from build123d import *

# Parameters (mm, degrees)
BOSS_EXTRUDE1_DEPTH  = 6
SKETCH3_W            = 26.265732208
SKETCH3_H            = 53.5
CUT_EXTRUDE2_DEPTH   = 6
BOSS_EXTRUDE2_DEPTH  = 3.175
CUT_EXTRUDE3_DEPTH   = 9.175
SKETCH5_W            = 6.5
SKETCH5_H            = 3
CUT_EXTRUDE4_DEPTH   = 6.95
SKETCH6_R            = 2.5
CUT_EXTRUDE5_DEPTH   = 10
M3_CLEARANCE_HOLE1_D = 3.2
SKETCH17_R           = 41
BOSS_EXTRUDE3_DEPTH  = 10
SKETCH18_R           = 2.5
CUT_EXTRUDE6_DEPTH   = 5
SKETCH19_R           = 4.5
CUT_EXTRUDE7_DEPTH   = 11.5
SKETCH20_R           = 2.706261539
SKETCH20_R_2         = 3.316969597
CUT_EXTRUDE8_DEPTH   = 6


with BuildPart() as part:
    # Sketch1 → Boss-Extrude1 (new body)
    with BuildSketch(Plane(origin=(0, 0, 0), x_dir=(1, 0, 0), z_dir=(0, 1, 0))):
        with BuildLine():
            Line((-21.25, 28.5), (-21.25, -28.5))
            ThreePointArc((-21.25, -28.5), (0, -33.5), (21.25, -28.5))
            Line((21.25, -28.5), (21.25, 28.5))
            Line((21.25, 28.5), (-21.25, 28.5))
        make_face()
        with BuildLine():
            Line((-17.45, 32), (-17.45, 28.5))
            Line((-17.45, 28.5), (17.45, 28.5))
            Line((17.45, 28.5), (17.45, 32))
            ThreePointArc((17.45, 32), (0, 37.8), (-17.45, 32))
        make_face()
    extrude(amount=BOSS_EXTRUDE1_DEPTH)

    # Sketch3 → Cut-Extrude2 (cut)
    with BuildSketch(Plane.XZ):
        with Locations((-30.582866104, -1.75)):
            Rectangle(SKETCH3_W, SKETCH3_H)
        with Locations((30.582866104, -1.75)):
            Rectangle(SKETCH3_W, SKETCH3_H)
    extrude(amount=-CUT_EXTRUDE2_DEPTH, mode=Mode.SUBTRACT)

    # Sketch2 → Boss-Extrude2 (add)
    with BuildSketch(Plane(origin=(0, 6, 0), x_dir=(1, 0, 0), z_dir=(0, 1, 0))):
        with BuildLine():
            Line((-7.375, 17.3), (-7.375, 37.8))
            Line((-7.375, 37.8), (7.375, 37.8))
            Line((7.375, 37.8), (7.375, 17.3))
            ThreePointArc((7.375, 17.3), (0, 12.5), (-7.375, 17.3))
        make_face()
    extrude(amount=BOSS_EXTRUDE2_DEPTH)

    # Sketch4 → Cut-Extrude3 (cut)
    with BuildSketch(Plane.XZ):
        with BuildLine():
            Line((17.45, -32), (17.45, -50.042511561))
            Line((17.45, -50.042511561), (-17.45, -50.042511561))
            Line((-17.45, -50.042511561), (-17.45, -32))
            ThreePointArc((-17.45, -32), (0, -37.8), (17.45, -32))
        make_face()
    extrude(amount=-CUT_EXTRUDE3_DEPTH, mode=Mode.SUBTRACT)

    # Sketch5 → Cut-Extrude4 (cut)
    with BuildSketch(Plane(origin=(0, 9.175, 0), x_dir=(1, 0, 0), z_dir=(0, 1, 0))):
        with Locations((0, 31.3)):
            Rectangle(SKETCH5_W, SKETCH5_H)
    extrude(amount=-CUT_EXTRUDE4_DEPTH, mode=Mode.SUBTRACT)

    # Sketch6 → Cut-Extrude5 (cut)
    with BuildSketch(Plane(origin=(0, 9.175, -37.8), x_dir=(-1, 0, 0), z_dir=(0, 0, -1))):
        with Locations((0, -4.2)):
            Circle(SKETCH6_R)
    extrude(amount=-CUT_EXTRUDE5_DEPTH, mode=Mode.SUBTRACT)

    # M3 Clearance Hole1 (through all)
    with Locations(Plane(origin=(0, 0, 0), x_dir=(-1, 0, 0), z_dir=(0, -1, 0))):
        with Locations((0, 2.15)):
            Hole(M3_CLEARANCE_HOLE1_D / 2)

    # Sketch17 → Boss-Extrude3 (add)
    with BuildSketch(Plane.XZ):
        with Locations((0, -2.15)):
            Circle(SKETCH17_R)
    extrude(amount=BOSS_EXTRUDE3_DEPTH)

    # Sketch18 → Cut-Extrude6 (cut)
    with BuildSketch(Plane.XZ.offset(10)):
        with Locations((17.78, -32.945863359)):
            Circle(SKETCH18_R)
        with Locations((35.56, -2.15)):
            Circle(SKETCH18_R)
        with Locations((17.78, 28.645863359)):
            Circle(SKETCH18_R)
        with Locations((-17.78, -32.945863359)):
            Circle(SKETCH18_R)
        with Locations((-35.56, -2.15)):
            Circle(SKETCH18_R)
        with Locations((-17.78, 28.645863359)):
            Circle(SKETCH18_R)
    extrude(amount=-CUT_EXTRUDE6_DEPTH, mode=Mode.SUBTRACT)

    # Sketch19 → Cut-Extrude7 (cut)
    with BuildSketch(Plane(origin=(0, 6, 0), x_dir=(1, 0, 0), z_dir=(0, 1, 0))):
        with Locations((-17.78, 32.945863359)):
            Circle(SKETCH19_R)
        with Locations((17.78, 32.945863359)):
            Circle(SKETCH19_R)
        with Locations((35.56, 2.15)):
            Circle(SKETCH19_R)
        with Locations((17.78, -28.645863359)):
            Circle(SKETCH19_R)
        with Locations((-17.78, -28.645863359)):
            Circle(SKETCH19_R)
        with Locations((-35.56, 2.15)):
            Circle(SKETCH19_R)
    extrude(amount=-CUT_EXTRUDE7_DEPTH, mode=Mode.SUBTRACT)

    # Sketch20 → Cut-Extrude8 (cut)
    with BuildSketch(Plane(origin=(0, 6, 0), x_dir=(1, 0, 0), z_dir=(0, 1, 0))):
        with Locations((-20.581445068, -26.580263628)):
            Circle(SKETCH20_R)
        with Locations((20.21362745, -26.580263628)):
            Circle(SKETCH20_R_2)
    extrude(amount=-CUT_EXTRUDE8_DEPTH, mode=Mode.SUBTRACT)


solid = part.part
Input: part model. Units: mm. Frame: model coordinates. A direction names the side the tool comes from. Coordinates: 2 decimals unless noted, no trailing zeros. Order: outer loops, then holes, each group sorted by start corner. A loop starts at its lowest first (then second) coordinate and runs counter-clockwise, first axis right, second up. Notation, with made-up numbers: M 72,4 L 94,4 A19 cw 94,34 Z; hole C 50.5,4 d11. An arc over 180 degrees is marked long. One line per question, with ' | ' between items.
Item 1: Section D-D (y = -1.25). Output: boundary loops of the cut face in (x, z), then the cut area to 3 significant figures.
Geometry results:
outline: C 0,-2.15 d82; hole C -35.56,-2.15 d9; hole C -17.78,-32.95 d9; hole C -17.78,28.65 d9; hole C 17.78,-32.95 d9; hole C 17.78,28.65 d9; hole C 35.56,-2.15 d9 | area: 4,900 mm^2
Item 2: Section A-A (z = -2.15). Output: boundary loops of the cut face in (x, y).
Geometry results:
outline: M -41,-10 L -38.06,-10 L -38.06,-5.5 L -40.06,-5.5 L -40.06,0 L -41,0 Z; M -33.06,-10 L 33.06,-10 L 33.06,-5.5 L 31.06,-5.5 L 31.06,0 L 17.45,0 L 17.45,6 L 1.6,6 L 1.6,0 L -1.6,0 L -1.6,6 L -17.45,6 L -17.45,0 L -31.06,0 L -31.06,-5.5 L -33.06,-5.5 Z; M 38.06,-10 L 41,-10 L 41,0 L 40.06,0 L 40.06,-5.5 L 38.06,-5.5 Z
Item 3: Pin query (flat end, axial travel): pin 1 (1.5 mm diameter, centred on x = 7.5, z = -21, fed in from +Y) (3 decimals); pin 2 (8 mm diameter, centred on x = 32.5, z = 22, fed in from +Y); pin 3 (6 mm diameter, centred on x = 20, y = 4, fed in from -Z); pin 4 (0.9 mm diameter, centred on y = 4.5, z = -31.5, fed in from +X). Return the tip coordinate at first contact, or that it passes through.
Geometry results:
pin 1: stops at y = 9.175 | pin 2: stops at y = 0 | pin 3: stops at z = -28.51 | pin 4: stops at x = 13.7
Item 4: Ray query, line 1 along Z through (x, y) = (0, 2.8); line 2 along Y through (x, z) = (0, -28.95) (3 decimals); line 3 along Z through (x, y) = (-17.78, -2.5). Return the intervals inside material, ascending.
Geometry results:
line 1: z = -27.8 to -3.75, -0.55 to 33.5 | line 2: y = -10 to 2.475, 7.475 to 9.175 | line 3: z = -39.09 to -37.45, -28.45 to 24.15, 33.15 to 34.79
Item 5: Reachability of faces 4 (the cylindrical face through (0.1, 7.6, -12.5)), 5 (the cylindrical face through (14.209, -0.947, -30.208)), 6 (the cylindrical face through (-0.2, 1.5, -37.8)), 7 (the cylindrical face through (0.325, 7.454, -35.335)) from +Z, -Z, +X, -X, +Y, -Y: full face, straight path, thin tool, end or side. Return the list, or none.
Geometry results:
face 4: +Z, +Y | face 5: +Y | face 6: -Z, +Y | face 7: -Z
Item 6: Section B-B (x = 0). Output: boundary loops of the cut face in (y, z) (3 decimals), then the cut area to 3 significant figures.
Geometry results:
outline: M -10,-43.15 L 0,-43.15 L 0,-37.8 L 2.475,-37.8 L 2.475,-32.8 L 2.225,-32.8 L 2.225,-29.8 L 2.475,-29.8 L 2.475,-27.8 L 7.475,-27.8 L 7.475,-29.8 L 9.175,-29.8 L 9.175,-12.5 L 6,-12.5 L 6,-3.75 L 0,-3.75 L 0,-0.55 L 6,-0.55 L 6,33.5 L 0,33.5 L 0,38.85 L -10,38.85 Z; M 7.475,-37.8 L 9.175,-37.8 L 9.175,-32.8 L 7.475,-32.8 Z | area: 1,250 mm^2
Item 7: Section C-C (x = 18.5). Output: boundary loops of the cut face in (y, z).
Geometry results:
outline: M -10,-38.74 L 0,-38.74 L 0,-37.39 L -5.5,-37.39 L -5.5,-35.34 L -10,-35.34 Z; M -10,-30.55 L -5.5,-30.55 L -5.5,-28.5 L 0,-28.5 L 0,24.2 L -5.5,24.2 L -5.5,26.25 L -10,26.25 Z; M -10,31.04 L -5.5,31.04 L -5.5,33.09 L 0,33.09 L 0,34.44 L -10,34.44 Z
Item 8: Draft query along Z for faces 1 (the cylindrical face through (32, -2.7, 0.6)), 2 (the cylindrical face through (37.874, -4.93, -17.853)), 3 (the flat face through (0, 9.175, -25)). Return one class per face: released by +Z, released by -Z, zero draft, split by the parting line, or undercut.
Geometry results:
face 1: undercut | face 2: split by the parting line | face 3: zero draft
